Autodesk Inventor part; units mm, degrees
ref_plane "YZ Plane" through (0, 0, 0) normal (1, 0, 0) x (0, 1, 0)
ref_plane "XZ Plane" through (0, 0, 0) normal (0, 1, 0) x (-1, 0, 0)
ref_plane "XY Plane" through (0, 0, 0) normal (0, 0, 1) x (1, 0, 0)
sketch "Sketch1" plane through (0, 0, 0) normal (0, 0, 1) x (1, 0, 0)
  line L0 (0, 0) -> (160, 0)
  line L1 (160, 0) -> (160, 140)
  line L2 (160, 140) -> (0, 140)
  line L3 (0, 140) -> (0, 0)
  line L4 (5, 135) -> (155, 135)
  line L5 (155, 135) -> (155, 5)
  line L6 (155, 5) -> (5, 5)
  line L7 (5, 5) -> (5, 135)
  dimension "d0" = 160
  dimension "d1" = 140
  dimension "d2" = 5
extrude "Extrusion1" add sketch "Sketch1" along normal blind 110
sketch "Sketch2" plane through (0, 0, 110) normal (0, 0, 1) x (1, 0, 0)
  line L0 (160, 0) -> (160, 140)
  line L1 (160, 140) -> (0, 140)
  line L2 (0, 140) -> (0, 0)
  line L3 (0, 0) -> (160, 0)
  line L4 (5, 135) -> (155, 135)
  line L5 (155, 135) -> (155, 5)
  line L6 (155, 5) -> (5, 5)
  line L7 (5, 5) -> (5, 135)
extrude "Extrusion2" add sketch "Sketch2" against normal blind 5 contours L4 L5 L6 L7
sketch "Sketch4" plane through (160, 0, 0) normal (1, 0, 0) x (0, 0, -1)
  line L0 (0, 0) -> (0, 140)
  line L1 (0, 140) -> (-110, 140)
  line L2 (-110, 0) -> (-110, 140)
  line L3 (0, 0) -> (-110, 0)
  line L4 (-110, 140) -> (-110, 130)
  line L5 (-110, 130) -> (-88, 130)
  line L6 (-88, 130) -> (-38, 130)
  line L7 (-38, 130) -> (-38, 105)
  line L8 (-38, 105) -> (-88, 105)
  line L9 (-88, 105) -> (-88, 130)
  point P0 (0, 0)
  dimension "d7" = 10
  dimension "d8" = 22
  dimension "d9" = 50
  dimension "d10" = 25
extrude "Extrusion3" cut sketch "Sketch4" against normal blind 5 contours L6 L7 L8 L9
sketch "Sketch5" plane through (0, 0, 110) normal (0, 0, 1) x (1, 0, 0)
  line L0 (160, 0) -> (160, 140)
  line L1 (160, 140) -> (0, 140)
  line L2 (0, 140) -> (0, 0)
  line L3 (0, 0) -> (160, 0)
  line L4 (80, 140) -> (80, 90)
  line L5 (80, 90) -> (30, 90)
  line L6 (30, 90) -> (30, 17)
  line L7 (30, 17) -> (80, 17)
  line L8 (80, 17) -> (80, 90)
  line L9 (80, 90) -> (130, 90)
  line L10 (130, 90) -> (130, 17)
  line L11 (130, 17) -> (80, 17)
  line L12 (130, 17) -> (120, 17)
  line L13 (120, 17) -> (120, 27)
  circle A0 centre (120, 27) radius 2.5
  line L14 (130, 53.5) -> (125, 53.5)
  circle A1 centre (40, 27) radius 2.5
  circle A2 centre (120, 80) radius 2.5
  circle A3 centre (40, 80) radius 2.5
  dimension "d13" = 50
  dimension "d14" = 50
  dimension "d15" = 73
  dimension "d16" = 10
  dimension "d17" = 10
  dimension "d18" = 5
  dimension "d19" = 5
extrude "Extrusion4" cut sketch "Sketch5" against normal blind 5 contours A0 | A1 | A2 | A3
sketch "Sketch6" plane through (0, 0, 110) normal (0, 0, 1) x (1, 0, 0)
  circle A0 centre (120, 80) radius 2.5
  circle A1 centre (40, 27) radius 2.5
  circle A2 centre (40, 80) radius 2.5
  circle A3 centre (120, 27) radius 2.5
  line L0 (160, 0) -> (160, 140)
  line L1 (160, 140) -> (0, 140)
  line L2 (0, 140) -> (0, 0)
  line L3 (0, 0) -> (160, 0)
  line L4 (160, 0) -> (141.053, 0)
  line L5 (0, 0) -> (160, 0)
  line L6 (141.053, 0) -> (141.053, 34.149)
  circle A4 centre (141.053, 34.149) radius 1
  line L7 (0, 140) -> (64.087, 140)
  line L8 (64.087, 140) -> (64.087, 83.191)
  circle A5 centre (64.087, 83.191) radius 1
  dimension "d22" = 18.947
  dimension "d23" = 34.149
  dimension "d24" = 2
  dimension "d28" = 64.087
  dimension "d29" = 56.809
  dimension "d30" = 2
extrude "Extrusion5" cut sketch "Sketch6" against normal blind 5 contours A5 | A4
fillet "Fillet1" radius 5 8 edges at (160, 0, 55) (0, 0, 55) (160, 140, 55) (0, 140, 55) (80, 0, 110) (0, 70, 110) (80, 140, 110) (160, 70, 110)
sketch "Sketch7" plane through (0, 0, 0) normal (0, 0, -1) x (-1, 0, 0)
  line L0 (-5, 135) -> (-155, 135)
  line L1 (-5, 5) -> (-5, 135)
  line L2 (-155, 5) -> (-5, 5)
  line L3 (-155, 135) -> (-155, 5)
  arc A0 (0, 135) -> (-5, 140) centre (-5, 135) ccw
  line L4 (-155, 140) -> (-5, 140)
  arc A1 (-155, 140) -> (-160, 135) centre (-155, 135) ccw
  line L5 (-160, 5) -> (-160, 135)
  arc A2 (-160, 5) -> (-155, 0) centre (-155, 5) ccw
  line L6 (-5, 0) -> (-155, 0)
  arc A3 (-5, 0) -> (0, 5) centre (-5, 5) ccw
  line L7 (0, 135) -> (0, 5)
  line L8 (-5, 135) -> (-12.5, 135)
  line L9 (-12.5, 135) -> (-12.5, 127.5)
  line L10 (-12.5, 127.5) -> (-5, 127.5)
  line L11 (-5, 127.5) -> (-5, 135)
  circle A4 centre (-12.5, 127.5) radius 1.5
  line L12 (-80, 135) -> (-80, 130)
  line L13 (-5, 70) -> (-10, 70)
  circle A5 centre (-147.5, 127.5) radius 1.5
  circle A6 centre (-12.5, 12.5) radius 1.5
  circle A7 centre (-147.5, 12.5) radius 1.5
  circle A8 centre (-12.5, 127.5) radius 4.5
  line L14 (-5, 123) -> (-12.5, 123)
  line L15 (-5, 5) -> (-5, 135)
  line L16 (-17, 127.5) -> (-17, 135)
  circle A9 centre (-147.5, 127.5) radius 4.5
  line L17 (-155, 123) -> (-147.5, 123)
  line L18 (-143, 127.5) -> (-143, 135)
  circle A10 centre (-12.5, 12.5) radius 4.5
  line L19 (-5, 17) -> (-12.5, 17)
  line L20 (-17, 12.5) -> (-17, 5)
  circle A11 centre (-147.5, 12.5) radius 4.5
  line L21 (-143, 12.5) -> (-143, 5)
  line L22 (-155, 17) -> (-147.5, 17)
  point P0 (0, 0)
  dimension "d31" = 7.5
  dimension "d32" = 7.5
  dimension "d33" = 3
  dimension "d34" = 5
  dimension "d35" = 5
  dimension "d36" = 3
extrude "Extrusion6" add sketch "Sketch7" against normal blind 10 contours L1 L10 A8 L9 L0 | L9 A8 L16 L0 | L1 L14 A8 L10 | A8 L10 A4 L9 | L9 A4 L10 A8 | L18 A9 L17 L3 L0 | L1 L2 L20 A10 L19 | A9 | A10 | L22 A11 L21 L2 L3 | A11
sketch "Sketch8" plane through (0, 0, 110) normal (0, 0, 1) x (1, 0, 0)
  line L0 (155, 140) -> (5, 140)
  line L1 (80, 140) -> (80, 65)
  line L2 (80, 65) -> (65, 65)
  line L3 (65, 65) -> (65, 50)
  line L4 (65, 50) -> (80, 50)
  line L5 (80, 50) -> (80, 65)
  line L6 (80, 65) -> (95, 65)
  line L7 (95, 65) -> (95, 50)
  line L8 (95, 50) -> (80, 50)
  point P0 (0, 0)
  dimension "d39" = 75
  dimension "d40" = 15
  dimension "d41" = 15
extrude "Extrusion7" cut sketch "Sketch8" against normal blind 10
sketch "Sketch9" plane through (160, 5, 0) normal (1, 0, 0) x (0, 0, -1)
  line L0 (0, 135) -> (-105, 135)
  line L1 (-110, 130) -> (-110, 0)
  line L2 (-105, -5) -> (0, -5)
  line L3 (-52.5, 135) -> (-52.5, 45)
  circle A0 centre (-52.5, 45) radius 8
  dimension "d44" = 90
  dimension "d45" = 16
extrude "Extrusion8" cut sketch "Sketch9" against normal blind 10
properties part number "BoxIoT"
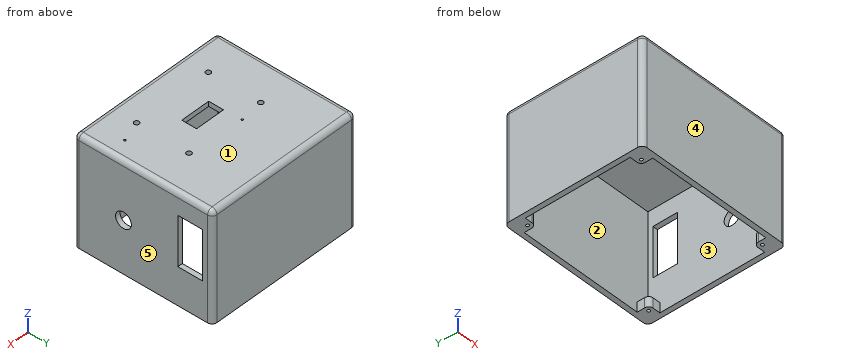
Check sheet for the modelled part. Datum: model origin and axes. Units: mm. Face numbers are marked on the shaded views. A direction names the side the tool comes from. Round coordinates to 2 decimals unless told otherwise and drop trailing zeros. Order: outer loops, then holes, each group sorted by start corner. A loop starts at its lowest first (then second) coordinate and runs counter-clockwise, first axis right, second up. Notation, with made-up numbers: (30.25, 42.25) - (70.25, 42.25) arc R8 cw to (70.25, 46.25) - close; hole circle Ø3 at (-28.5, 5). An arc over 180 degrees is marked (long way). Answer as CSV lines item,"result". Start each with the question number.
1) Tool access check on the marked faces 1 and 2. Record the directions out of +Z, -Z, +X, -X, +Y, -Y that give a thin tool (end or side, any length) a straight path to the whole face; none if there is none.
2) Scan lines: probe 1 along Y at (x, z) = (133.5, 31.5); probe 2 along X at (y, z) = (60, 5); probe 3 along Y at (x, z) = (12.5, 4). Record each from-to range of solid material in increasing order.
3) Section check D-D (y = 114.5). Record the cut outline in (x, z).
4) Draft check along X on the marked faces 3, 4 and 5. Enter one of: +X half, -X half, draft (parallel to the pull), parting line (faces both ways), or undercut.
5) Section check C-C (y = 80). Record the cut outline in (x, z).
6) Section check A-A (z = 52.5). Record the cut outline in (x, y).
7) Section check B-B (x = 120). Record the cut outline in (y, z), then the cut area to 3 significant figures.
8) Depth check by flat-ended pin: pin 1 (8 mm diameter, centred on x = 54.5, y = 125, fed in from -Z); pin 2 (3 mm diameter, centred on x = 40, y = 27, fed in from -Z); pin 3 (2.5 mm diameter, centred on y = 58, z = 107.5, fed in from +X). Enter the tip coordinate at first touch or a pass-through.
Determined:
1,face 1,"+Z, +X, -X, +Y, -Y"
1,face 2,"none"
2,probe 1,"0 to 5, 135 to 140"
2,probe 2,"0 to 5, 155 to 160"
2,probe 3,"0 to 11, 14 to 17, 123 to 126, 129 to 140"
3,outline,"(0, 0) - (5, 0) - (5, 105) - (155, 105) - (155, 88) - (160, 88) - (160, 105) arc R5 ccw to (155, 110) - (5, 110) arc R5 ccw to (0, 105) - close; (155, 0) - (160, 0) - (160, 38) - (155, 38) - close"
4,face 3,"undercut"
4,face 4,"draft"
4,face 5,"+X half"
5,outline,"(0, 0) - (5, 0) - (5, 105) - (37.5, 105) - (37.5, 110) - (5, 110) arc R5 ccw to (0, 105) - close; (42.5, 105) - (117.5, 105) - (117.5, 110) - (42.5, 110) - close; (122.5, 105) - (155, 105) - (155, 0) - (160, 0) - (160, 105) arc R5 ccw to (155, 110) - (122.5, 110) - close"
6,outline,"(0, 5) arc R5 ccw to (5, 0) - (155, 0) arc R5 ccw to (160, 5) - (160, 42) - (155, 42) - (155, 5) - (5, 5) - (5, 135) - (155, 135) - (155, 130) - (160, 130) - (160, 135) arc R5 ccw to (155, 140) - (5, 140) arc R5 ccw to (0, 135) - close; (155, 58) - (160, 58) - (160, 105) - (155, 105) - close"
7,outline,"(0, 0) - (5, 0) - (5, 105) - (24.5, 105) - (24.5, 110) - (5, 110) arc R5 ccw to (0, 105) - close; (29.5, 105) - (77.5, 105) - (77.5, 110) - (29.5, 110) - close; (82.5, 105) - (135, 105) - (135, 0) - (140, 0) - (140, 105) arc R5 ccw to (135, 110) - (82.5, 110) - close"
7,area,"1,690 mm^2"
8,pin 1,"z = 105"
8,pin 2,"through"
8,pin 3,"x = 159.84"
